```python
from build123d import *

# Parameters (mm, degrees)
F0_R     = 13.3135020733
F0_R_2   = 14.2906457186
F1_DEPTH = 15.4849458486
F2_W     = 54.254218936
F2_H     = 18.4195190668
F3_DEPTH = 25.4
F4_R     = 5.08
F5_DEPTH = 25.4
F6_W     = 46.2679080665
F6_H     = 42.419552803
F7_DEPTH = 13.794451952


# Not quite as in the source:
# - the program builds the solid bodies; features that only make, move or delete a surface that nothing else refers to are left out


with BuildPart() as f1:
    # F0 (on Front) → F1 (new body)
    with BuildSketch(Plane.XZ):
        with BuildLine():
            Line((47.7382689714, 29.4530540705), (-48.2266321778, 29.4530540705))
            ThreePointArc((-48.2266321778, 29.4530540705), (-77.6628926396, 0.0167936087), (-48.2266321778, -29.4194668531))
            Line((-48.2266321778, -29.4194668531), (47.7382689714, -29.4194668531))
            ThreePointArc((47.7382689714, -29.4194668531), (77.1745294333, 0.0167936087), (47.7382689714, 29.4530540705))
        make_face()
        with Locations((-48.2266321778, 0.0167936087)):
            Circle(F0_R, mode=Mode.SUBTRACT)
        with Locations((47.7382689714, 0.0167936087)):
            Circle(F0_R_2, mode=Mode.SUBTRACT)
    extrude(amount=F1_DEPTH)

    # F2 (on Front) → F3 (join)
    with BuildSketch(Plane.XZ):
        with Locations((-2.6991143823, 21.6291323304)):
            Rectangle(F2_W, F2_H)
    extrude(amount=F3_DEPTH)

    # F4
    f4_edges = [f1.edges().sort_by_distance(p)[0] for p in [
        (-2.699114, -25.4, 30.838892),
    ]]
    fillet(f4_edges, radius=F4_R)

    # F5 (add): a face of the model
    f5_faces = [f1.faces().sort_by_distance(p)[0] for p in [
        (-2.6991143823, -25.4, 19.0891323304),
    ]]
    extrude(f5_faces, amount=F5_DEPTH)

    # F6 (on Right) → F7 (join)
    with BuildSketch(Plane.YZ):
        with Locations((-23.1339540333, 4.6068131924)):
            Rectangle(F6_W, F6_H)
    extrude(amount=-F7_DEPTH)


solid = f1.part
```
Read the model definition and answer for the solid it produces. Units are mm, in the model's axes. A direction names the side the tool comes from. Give positions to 0.01 mm unless a question says otherwise; leave off trailing zeros. Write each loop counter-clockwise with the first axis right and the second up, starting at its lowest first coordinate (ties: lowest second). Pieces come first, ordered by that corner, then holes. Notation, with made-up numbers: (28.5, 10.5) - (69.5, 10.5) arc R20 cw to (69.5, 33.5) - close; hole circle Ø7 at (14.5, 1). An arc over 180 degrees is marked (long way). Write item = value, one per line. Start each with the question number.
Item 1: The mould has two halves that part along X. Classify faces 4 (the cylindrical face through (-77.656, -7.634, 0.664)), 5 (the flat face through (3, -38, 25.759)), 6 (the cylindrical face through (33.46, -7.63, 0.65)): +X half, -X half, draft (parallel to the pull), parting line (faces both ways), or undercut.
Item 2: Find section D-D (x = 57.5). Give the vertices of the cut face in (y, z), then the cut area to 3 significant figures.
Item 3: Find section C-C (y = -31). Give the vertices of the cut face in (x, z).
Item 4: Each of these flat-tipped pins is pushed along its axis until it touches: P1, Ø7.5, axis at x = -7, y = -44.5, coming from the +Z side; P2, Ø5, axis at y = -26, z = 8.5, coming from the +X side; P3, Ø1.5, axis at y = -33.5, z = -16, coming from the -X side; P4, Ø4, axis at x = -37, z = 20, coming from the +Y side. Where does it stop, or does it pass through?
Item 5: Find section B-B (z = -2.5). Give the vertices of the cut face in (x, y).
Item 6: A tool of negligible diameter and unlimited length cuts with its end or side. For faces 1 (the flat face through (-7, -31, -16.603)), 2 (the flat face through (36, -8, 29.453)), 3 (the flat face through (0, -31, -2)), from which of +Z, -Z, +X, -X, +Y, -Y can it reach the whole face along a straight path? Write none if from no direction.
Item 7: Find the intervals of material crossed by probe 1 along Y at (x, z) = (-6.5, -22); probe 2 along X at (y, z) = (-23.5, -3); probe 3 along Z at (x, y) = (-6, -35), in increasing order. Write a range as [from, to].
Item 8: Find section A-A (x = -7). Give the vertices of the cut face in (y, z), then the cut area to 3 significant figures.
Response:
q1.face_4 = -X half
q1.face_5 = draft
q1.face_6 = undercut
q2.outline = (-15.48, -27.75) - (0, -27.75) - (0, -10.42) - (-15.48, -10.42) - close; (-15.48, 10.45) - (0, 10.45) - (0, 27.79) - (-15.48, 27.79) - close
q2.area = 537 mm²
q3.outline = (-29.83, 12.42) - (-13.79, 12.42) - (-13.79, -16.6) - (0, -16.6) - (0, 12.42) - (24.43, 12.42) - (24.43, 25.76) - (0, 25.76) - (0, 25.82) - (-13.79, 25.82) - (-13.79, 25.76) - (-29.83, 25.76) - close
q4.P1 = 25.82
q4.P2 = 0
q4.P3 = -13.79
q4.P4 = 0
q5.outline = (-77.56, -15.48) - (-61.3, -15.48) - (-61.3, 0) - (-77.56, 0) - close; (-35.15, -15.48) - (-13.79, -15.48) - (-13.79, -46.27) - (0, -46.27) - (0, -15.48) - (33.67, -15.48) - (33.67, 0) - (-35.15, 0) - close; (61.81, -15.48) - (77.07, -15.48) - (77.07, 0) - (61.81, 0) - close
q6.face_1 = -Z, +X, -X, -Y
q6.face_2 = +Z, +X, +Y, -Y
q6.face_3 = -Z, +X, -Y
q7.probe_1 = [-15.48, 0]
q7.probe_2 = [-13.79, 0]
q7.probe_3 = [-16.6, 25.82]
q8.outline = (-50.8, 12.42) - (-46.27, 12.42) - (-46.27, -16.6) - (-15.48, -16.6) - (-15.48, -29.42) - (0, -29.42) - (0, 30.84) - (-20.32, 30.84) arc R5.08 ccw to (-25.4, 25.82) - (-46.27, 25.82) - (-46.27, 25.76) - (-50.8, 25.76) - close
q8.area = 2,340 mm²
